Geometry check sheet. Reference: the model listing, model coordinates, mm. A direction names the side the tool comes from. Coordinates: 2 decimals unless noted, no trailing zeros. Loops run counter-clockwise (first coordinate to the right, second up) from the corner with the lowest first, then second, coordinate; pieces in that order, holes last. Notation, with made-up numbers: (-1, 78) -> (44, 78) arc R13 ccw to (44, 84) -> close; hole circle Ø8 at (22, 64). An arc over 180 degrees is marked (long way). Answer as a JSON object with one key per item and string values.
from build123d import *

# Parameters (mm, degrees)
CROQUIS1_W                   = 47.6
CROQUIS1_H                   = 47.6
SALIENTE_EXTRUIR1_DEPTH      = 30
SALIENTE_EXTRUIR2_DEPTH      = 25
SALIENTE_EXTRUIR2_DEPTH_BACK = 25
CROQUIS3_R                   = 4
CORTAR_EXTRUIR1_DEPTH        = 63.501519982
CROQUIS4_R                   = 2.5
CROQUIS4_R_2                 = 3.5
CORTAR_EXTRUIR2_DEPTH        = 63.501519982
CHAFL_N1_SIZE                = 1


with BuildPart() as part:
    # Croquis1 → Saliente-Extruir1 (new body)
    with BuildSketch(Plane.XY):
        Rectangle(CROQUIS1_W, CROQUIS1_H)
    extrude(amount=SALIENTE_EXTRUIR1_DEPTH)

    # Croquis2 → Saliente-Extruir2 (add, two sides: drawn at the far end of the back side and taken through both)
    with BuildSketch(Plane(origin=(0, 0, 0), x_dir=(1, 0, 0), z_dir=(0, 1, 0)).offset(-SALIENTE_EXTRUIR2_DEPTH_BACK)):
        with BuildLine():
            Line((-25, 0), (25, 0))
            ThreePointArc((25, 0), (0, 13.232432916), (-25, 0))
        make_face()
    extrude(amount=SALIENTE_EXTRUIR2_DEPTH + SALIENTE_EXTRUIR2_DEPTH_BACK)

    # Croquis3 → Cortar-Extruir1 (cut, through all)
    with BuildSketch(Plane(origin=(0, 23.8, 0), x_dir=(1, 0, 0), z_dir=(0, 1, 0))):
        with Locations(Location((0, -17, 0), (0, 0, 270))):
            Circle(CROQUIS3_R)
    extrude(amount=-CORTAR_EXTRUIR1_DEPTH, mode=Mode.SUBTRACT)

    # Croquis4 → Cortar-Extruir2 (cut, through all)
    with BuildSketch(Plane(origin=(23.8, 0, 0), x_dir=(0, 0, -1), z_dir=(1, 0, 0))):
        with Locations(Location((-10, 19, 0), (0, 0, 90))):
            Circle(CROQUIS4_R)
        with Locations(Location((-25, 19, 0), (0, 0, 90))):
            Circle(CROQUIS4_R)
        with Locations(Location((-25, -19, 0), (0, 0, 90))):
            Circle(CROQUIS4_R)
        with Locations(Location((-10, -19, 0), (0, 0, 90))):
            Circle(CROQUIS4_R)
        with Locations(Location((-17, 0, 0), (0, 0, 90))):
            Circle(CROQUIS4_R_2)
    extrude(amount=-CORTAR_EXTRUIR2_DEPTH, mode=Mode.SUBTRACT)

    # Chaflán1
    chafl_n1_edges = [part.edges().sort_by_distance(p)[0] for p in [
        (-23.8, 0, 30),
        (0, -23.8, 30),
        (23.8, 0, 30),
        (0, 23.8, 30),
    ]]
    chamfer(chafl_n1_edges, length=CHAFL_N1_SIZE)


solid = part.part
1. Mould release check, pull along Z, two halves, no side actions. Record for faces 6 (the face through (0.3, -21, 8.5)), 7 (the face through (0, 0, 30)), 8 (the face through (-23.8, 0, 11)): released by +Z, released by -Z, zero draft, split by the parting line, or undercut.
Evaluation:
{"face 6": "undercut", "face 7": "released by +Z", "face 8": "zero draft"}
2. Thickness scan on probe 1 along Z at (x, y) = (5.5, 17); probe 2 along Y at (x, z) = (9, 17); probe 3 along X at (y, z) = (11, 2.5). Record the ranges inside material, lowest first. Write a range as from..to.
Evaluation:
{"probe 1": "z = -12.73..8.5, 11.5..23.5, 26.5..30", "probe 2": "y = -23.8..-3.5, 3.5..23.8", "probe 3": "x = -23.8..23.8"}
3. Section check C-C, the plane x = 1. Record the boundary of the cut face in (y, z).
Evaluation:
{"outline": "(-25, -13.22) -> (25, -13.22) -> (25, 0) -> (23.8, 0) -> (23.8, 13.13) -> (-23.8, 13.13) -> (-23.8, 0) -> (-25, 0) -> close; (-23.8, 20.87) -> (23.8, 20.87) -> (23.8, 29) -> (22.8, 30) -> (-22.8, 30) -> (-23.8, 29) -> close; hole circle Ø5 at (-19, 10); hole circle Ø5 at (-19, 25); hole circle Ø5 at (19, 10); hole circle Ø5 at (19, 25)"}
4. Depth check by flat-ended pin: P1, Ø1, axis at y = 15, z = 10, coming from the -X side; P2, Ø8, axis at x = 1, z = 21.5, coming from the -Y side; P3, Ø2, axis at x = -9, z = 8.5, coming from the +Y side. Enter the tip coordinate at first touch or a pass-through.
Evaluation:
{"P1": "stops at x = -23.8", "P2": "stops at y = -23.8", "P3": "stops at y = 23.8"}
5. Section check A-A, the plane y = -19. Record the boundary of the cut face in (x, z).
Evaluation:
{"outline": "(-25, 0) arc R30.23 ccw to (25, 0) -> (23.8, 0) -> (23.8, 7.5) -> (-23.8, 7.5) -> (-23.8, 0) -> close; (-23.8, 12.5) -> (23.8, 12.5) -> (23.8, 22.5) -> (-23.8, 22.5) -> close; (-23.8, 27.5) -> (23.8, 27.5) -> (23.8, 29) -> (22.8, 30) -> (-22.8, 30) -> (-23.8, 29) -> close; hole circle Ø8 at (0, 17)"}
6. Section check B-B, the plane z = 17. Record the boundary of the cut face in (x, y), then the cut area to 3 significant figures.
Evaluation:
{"outline": "(-23.8, -23.8) -> (-4, -23.8) -> (-4, -3.5) -> (-23.8, -3.5) -> close; (-23.8, 3.5) -> (-4, 3.5) -> (-4, 23.8) -> (-23.8, 23.8) -> close; (4, -23.8) -> (23.8, -23.8) -> (23.8, -3.5) -> (4, -3.5) -> close; (4, 3.5) -> (23.8, 3.5) -> (23.8, 23.8) -> (4, 23.8) -> close", "area": "1,610 mm^2"}
7. Section check D-D, the plane z = 25. Record the boundary of the cut face in (x, y), then the cut area to 3 significant figures.
Evaluation:
{"outline": "(-23.8, -23.8) -> (23.8, -23.8) -> (23.8, -21.5) -> (-23.8, -21.5) -> close; (-23.8, -16.5) -> (23.8, -16.5) -> (23.8, 16.5) -> (-23.8, 16.5) -> close; (-23.8, 21.5) -> (23.8, 21.5) -> (23.8, 23.8) -> (-23.8, 23.8) -> close", "area": "1,790 mm^2"}
8. Tool access check on faces 1 (the face through (0, 25, -5)), 2 (the face through (0.41, -0.35, -13.23)), 3 (the face through (0, -23.8, 11)), 4 (the face through (0, 23.8, 11)), 5 (the face through (23.8, 0, 11)). Record the directions out of +Z, -Z, +X, -X, +Y, -Y that give a thin tool (end or side, any length) a straight path to the whole face; none if there is none.
Evaluation:
{"face 1": "+Z, -Z, +X, -X, +Y", "face 2": "-Z, +Y, -Y", "face 3": "+Z, +X, -X, -Y", "face 4": "+Z, +X, -X, +Y", "face 5": "+Z, +X, +Y, -Y"}
